from build123d import *

# Parameters (mm, degrees)
SKETCH_1_W          = 20
SKETCH_1_H          = 60
EXTRUDE_1_DEPTH     = 8
EXTRUDE_2_DEPTH     = 4
SKETCH_4_W          = 10
SKETCH_4_H          = 60
EXTRUDE_3_DEPTH     = 4
SKETCH_5_R          = 2.5
CUT_EXTRUDE_1_DEPTH = 67
CUT_EXTRUDE_2_DEPTH = 10


with BuildPart() as part:
    # 草图1 → 凸台-拉伸1 (new body)
    with BuildSketch(Plane(origin=(0, 0, 0), x_dir=(1, 0, 0), z_dir=(0, 1, 0))):
        Rectangle(SKETCH_1_W, SKETCH_1_H)
    extrude(amount=EXTRUDE_1_DEPTH)

    # 草图3 → 凸台-拉伸2 (add)
    with BuildSketch(Plane(origin=(0, 8, 0), x_dir=(1, 0, 0), z_dir=(0, 1, 0))):
        Polygon((10, -30), (10, 30), (-50, 30), (-50, 20), (-10, 20), (-10, -20), (-50, -20), (-50, -30), align=None)
    extrude(amount=EXTRUDE_2_DEPTH)

    # 草图4 → 凸台-拉伸3 (add)
    with BuildSketch(Plane(origin=(0, 12, 0), x_dir=(1, 0, 0), z_dir=(0, 1, 0))):
        with Locations((-45, 0)):
            Rectangle(SKETCH_4_W, SKETCH_4_H)
    extrude(amount=-EXTRUDE_3_DEPTH)

    # 草图5 → 切除-拉伸1 (cut)
    with BuildSketch(Plane(origin=(0, 12, 0), x_dir=(1, 0, 0), z_dir=(0, 1, 0))):
        with Locations(Location((0, 15, 0), (0, 0, 270))):
            Circle(SKETCH_5_R)
        with Locations(Location((0, -15, 0), (0, 0, 270))):
            Circle(SKETCH_5_R)
    extrude(amount=-CUT_EXTRUDE_1_DEPTH, mode=Mode.SUBTRACT)

    # 草图7 → 切除-拉伸2 (cut)
    with BuildSketch(Plane.XZ.offset(-8)):
        with BuildLine():
            ThreePointArc((-21.275, 25), (-23.275, 27), (-25.275, 25))
            ThreePointArc((-25.275, 25), (-23.275, 23), (-21.275, 25))
        make_face()
        with BuildLine():
            ThreePointArc((-30.925, 25), (-32.925, 27), (-34.925, 25))
            ThreePointArc((-34.925, 25), (-32.925, 23), (-30.925, 25))
        make_face()
        with BuildLine():
            ThreePointArc((-25.275, -25), (-23.275, -27), (-21.275, -25))
            ThreePointArc((-21.275, -25), (-23.275, -23), (-25.275, -25))
        make_face()
        with BuildLine():
            ThreePointArc((-34.925, -25), (-32.925, -27), (-30.925, -25))
            ThreePointArc((-30.925, -25), (-32.925, -23), (-34.925, -25))
        make_face()
    extrude(amount=-CUT_EXTRUDE_2_DEPTH, mode=Mode.SUBTRACT)


solid = part.part
The model under review builds one solid part; all positions refer to its coordinate system, in mm. A direction names the side the tool comes from. Coordinates: 2 decimals unless noted, no trailing zeros. Write each loop counter-clockwise with the first axis right and the second up, starting at its lowest first coordinate (ties: lowest second). Pieces come first, ordered by that corner, then holes. Notation, with made-up numbers: (86.5, 60) - (96.5, 60) arc R13 cw to (96.5, 76) - close; hole circle Ø10 at (88.25, 5.5). An arc over 180 degrees is marked (long way). Answer as a JSON object with one key per item and string values. Group by question number.
1. Add section D-D (y = 10.75). Give the boundary of the cut face in (x, z) (3 decimals), plus the area to 3 significant figures.
2. Add section B-B (z = 18.5). Give the boundary of the cut face in (x, y).
3. Mouldability with a two-part tool opening along Z and no side actions: class faces 1 (the face through (-44, 8, -7)), 2 (the face through (-25.183, 9.972, 24.399)), 3 (the face through (-14, 9, 30)) as pulls with the +Z half, pulls with the -Z half, needs draft (parallel to the pull), parting line crosses it, or undercut.
4. Add section A-A (x = -26.5). Give the boundary of the cut face in (y, z).
5. Add section C-C (z = -25). Give the boundary of the cut face in (x, y) (3 decimals), plus the area to 3 significant figures.
6. Clearance check with a flat-ended pin moving along its axis: pin 1 Ø20 at (x, z) = (-31.5, 10.5) entering from -Y. State where the tip first meets the part, or that it passes through.
7. Machinability: for faces 4 (the face through (-25, 10, -20)), 5 (the face through (-10, 6, 0)), 6 (the face through (0, 0, 0)), which of the approach directions +Z, -Z, +X, -X, +Y, -Y give a long, thin tool a straight path to every point of the face, cutting with its end or side? Answer none if there is none.
8. To check wall thickness, follow probe 1 along Z at (x, y) = (-33, 8.5); probe 2 along X at (y, z) = (6.5, 15); probe 3 along Z at (x, y) = (-19, 11.25). State the ranges of each line that lie inside material, in increasing order.
Findings:
{
 "1": {"outline": "(-50, -30) - (10, -30) - (10, 30) - (-50, 30) - close; hole (-40, -20) - (-10, -20) - (-10, 20) - (-40, 20) - close; hole circle Ø4 at (-32.925, -25); hole circle Ø4 at (-32.925, 25); hole circle Ø4 at (-23.275, -25); hole circle Ø4 at (-23.275, 25); hole circle Ø5 at (0, -15); hole circle Ø5 at (0, 15)", "area": "2,310 mm²"},
 "2": {"outline": "(-50, 8) - (-40, 8) - (-40, 12) - (-50, 12) - close; (-10, 0) - (10, 0) - (10, 12) - (-10, 12) - close"},
 "3": {"face 1": "needs draft", "face 2": "undercut", "face 3": "pulls with the +Z half"},
 "4": {"outline": "(8, -30) - (12, -30) - (12, -20) - (8, -20) - close; (8, 20) - (12, 20) - (12, 30) - (8, 30) - close"},
 "5": {"outline": "(-50, 8) - (-34.925, 8) - (-34.925, 12) - (-50, 12) - close; (-30.925, 8) - (-25.275, 8) - (-25.275, 12) - (-30.925, 12) - close; (-21.275, 8) - (-10, 8) - (-10, 0) - (10, 0) - (10, 12) - (-21.275, 12) - close", "area": "368 mm²"},
 "6": {"pin 1": "y = 8"},
 "7": {"face 4": "+Y, -Y", "face 5": "-Y", "face 6": "+Z, -Z, +X, -X, -Y"},
 "8": {"probe 1": "-30 to -27, -23 to -20, 20 to 23, 27 to 30", "probe 2": "-10 to -2.5, 2.5 to 10", "probe 3": "-30 to -20, 20 to 30"}
}
